from build123d import *

# Parameters (mm, degrees)
SKETCH1_R           = 1.5
BOSS_EXTRUDE1_DEPTH = 1.75
BOSS_EXTRUDE2_DEPTH = 3
BOSS_EXTRUDE3_DEPTH = 0.5
SKETCH4_R           = 0.26
CUT_EXTRUDE1_DEPTH  = 42.78890403


with BuildPart() as part:
    # Sketch1 → Boss-Extrude1 (new body)
    with BuildSketch(Plane(origin=(0, 0, 0), x_dir=(1, 0, 0), z_dir=(0, 1, 0))):
        with BuildLine():
            Line((-18, 20), (18, 20))
            ThreePointArc((18, 20), (19.414213562, 19.414213562), (20, 18))
            Line((20, 18), (20, -18))
            ThreePointArc((20, -18), (19.414213562, -19.414213562), (18, -20))
            Line((18, -20), (-18, -20))
            ThreePointArc((-18, -20), (-19.414213562, -19.414213562), (-20, -18))
            Line((-20, -18), (-20, 18))
            ThreePointArc((-20, 18), (-19.414213562, 19.414213562), (-18, 20))
        make_face()
        with Locations(Location((-15.25, 15.25, 0), (0, 0, 270))):
            Circle(SKETCH1_R, mode=Mode.SUBTRACT)
        with Locations(Location((15.25, 15.25, 0), (0, 0, 270))):
            Circle(SKETCH1_R, mode=Mode.SUBTRACT)
        with Locations(Location((15.25, -15.25, 0), (0, 0, 270))):
            Circle(SKETCH1_R, mode=Mode.SUBTRACT)
        with Locations(Location((-15.25, -15.25, 0), (0, 0, 270))):
            Circle(SKETCH1_R, mode=Mode.SUBTRACT)
    extrude(amount=BOSS_EXTRUDE1_DEPTH)

    # Sketch2 → Boss-Extrude2 (add)
    with BuildSketch(Plane.XY.offset(20)):
        with BuildLine():
            Line((7.26, 1.75), (7.26, 2.78))
            ThreePointArc((7.26, 2.78), (7.318578644, 2.921421356), (7.46, 2.98))
            Line((7.46, 2.98), (7.705, 2.98))
            ThreePointArc((7.705, 2.98), (7.846421356, 3.038578644), (7.905, 3.18))
            Line((7.905, 3.18), (7.905, 3.55))
            ThreePointArc((7.905, 3.55), (7.963578644, 3.691421356), (8.105, 3.75))
            Line((8.105, 3.75), (10.415, 3.75))
            ThreePointArc((10.415, 3.75), (10.556421356, 3.691421356), (10.615, 3.55))
            Line((10.615, 3.55), (10.615, 3.18))
            ThreePointArc((10.615, 3.18), (10.673578644, 3.038578644), (10.815, 2.98))
            Line((10.815, 2.98), (11.06, 2.98))
            ThreePointArc((11.06, 2.98), (11.201421356, 2.921421356), (11.26, 2.78))
            Line((11.26, 2.78), (11.26, 1.75))
            Line((11.26, 1.75), (7.26, 1.75))
        make_face()
        with BuildLine():
            Line((7.36, 1.85), (7.36, 2.78))
            ThreePointArc((7.36, 2.78), (7.389289322, 2.850710678), (7.46, 2.88))
            Line((7.46, 2.88), (7.705, 2.88))
            ThreePointArc((7.705, 2.88), (7.917132034, 2.967867966), (8.005, 3.18))
            Line((8.005, 3.18), (8.005, 3.55))
            ThreePointArc((8.005, 3.55), (8.034289322, 3.620710678), (8.105, 3.65))
            Line((8.105, 3.65), (10.415, 3.65))
            ThreePointArc((10.415, 3.65), (10.485710678, 3.620710678), (10.515, 3.55))
            Line((10.515, 3.55), (10.515, 3.18))
            ThreePointArc((10.515, 3.18), (10.602867966, 2.967867966), (10.815, 2.88))
            Line((10.815, 2.88), (11.06, 2.88))
            ThreePointArc((11.06, 2.88), (11.130710678, 2.850710678), (11.16, 2.78))
            Line((11.16, 2.78), (11.16, 1.85))
            Line((11.16, 1.85), (7.36, 1.85))
        make_face(mode=Mode.SUBTRACT)
    extrude(amount=-BOSS_EXTRUDE2_DEPTH)

    # Sketch3 → Boss-Extrude3 (add)
    with BuildSketch(Plane(origin=(0, 0, 17), x_dir=(-1, 0, 0), z_dir=(0, 0, -1))):
        with BuildLine():
            Line((-11.26, 1.75), (-7.26, 1.75))
            Line((-7.26, 1.75), (-7.26, 2.78))
            ThreePointArc((-7.26, 2.78), (-7.318578644, 2.921421356), (-7.46, 2.98))
            Line((-7.46, 2.98), (-7.705, 2.98))
            ThreePointArc((-7.705, 2.98), (-7.846421356, 3.038578644), (-7.905, 3.18))
            Line((-7.905, 3.18), (-7.905, 3.55))
            ThreePointArc((-7.905, 3.55), (-7.963578644, 3.691421356), (-8.105, 3.75))
            Line((-8.105, 3.75), (-10.415, 3.75))
            ThreePointArc((-10.415, 3.75), (-10.556421356, 3.691421356), (-10.615, 3.55))
            Line((-10.615, 3.55), (-10.615, 3.18))
            ThreePointArc((-10.615, 3.18), (-10.673578644, 3.038578644), (-10.815, 2.98))
            Line((-10.815, 2.98), (-11.06, 2.98))
            ThreePointArc((-11.06, 2.98), (-11.201421356, 2.921421356), (-11.26, 2.78))
            Line((-11.26, 2.78), (-11.26, 1.75))
        make_face()
    extrude(amount=BOSS_EXTRUDE3_DEPTH)

    # Sketch4 → Cut-Extrude1 (cut, through all)
    with BuildSketch(Plane(origin=(0, 0, 16.5), x_dir=(-1, 0, 0), z_dir=(0, 0, -1))):
        with Locations((-10.2, 2.87)):
            Circle(SKETCH4_R)
        with Locations((-9.3, 2.87)):
            Circle(SKETCH4_R)
        with Locations((-8.4, 2.87)):
            Circle(SKETCH4_R)
    extrude(amount=-CUT_EXTRUDE1_DEPTH, mode=Mode.SUBTRACT)


solid = part.part
Source: CAD feature listing. Evaluate the final solid. Frame: model axes, mm. A direction names the side the tool comes from. Coordinates: 2 decimals unless noted, no trailing zeros. Order: outer loops, then holes, each group sorted by start corner. A loop starts at its lowest first (then second) coordinate and runs counter-clockwise, first axis right, second up. Notation, with made-up numbers: M 59.25,-26 L 76.25,-26 A11 cw 76.25,-12 Z; hole C 4,16.25 d10. An arc over 180 degrees is marked long. Write each question's results on one line, items separated by ' | '. Start each with the question number.
1. Section D-D, the plane x = 3.5. Return the cut outline in (y, z), then the cut area to 3 significant figures.
2. Draft query along Y for faces 1 (the face through (-20, 1, 0)), 2 (the face through (0, 0, 0)), 3 (the face through (9, 1.85, 19)). Return one class per face: +Y half, -Y half, draft (parallel to the pull), parting line (faces both ways), or undercut.
3. Section B-B, the plane z = -15.25. Return the cut outline in (x, y).
4. Reachability of faces 4 (the face through (9, 2, 16.5)), 5 (the face through (-15.18, 0.86, -16.75)) from +Z, -Z, +X, -X, +Y, -Y: full face, straight path, thin tool, end or side. Return the list, or none.
5. Section C-C, the plane y = 0.8. Return the cut outline in (x, z), then the cut area to 3 significant figures.
6. Section A-A, the plane x = 15.25. Return the cut outline in (y, z).
7. Material intervals for L1, parallel to X at y = 1.05, z = 15.25; L2, parallel to Y at x = 9.3, z = 16.6; L3, parallel to Y at x = 10, z = 6.5, sorted ascending.
8. Pin query (flat end, axial travel): pin 1 (1 mm diameter, centred on x = 9, y = 2.5, fed in from -Z); pin 2 (3 mm diameter, centred on x = -13.5, z = -6.5, fed in from -Y); pin 3 (0.8 mm diameter, centred on y = 2.5, z = 19, fed in from -X); pin 4 (8 mm diameter, centred on x = -14, z = 3.5, fed in from +Y). Return the tip coordinate at first contact, or that it passes through.
Solution:
1) outline: M 0,-20 L 1.75,-20 L 1.75,20 L 0,20 Z | area: 70.0 mm²
2) face 1: draft | face 2: -Y half | face 3: undercut
3) outline: M -20,0 L -16.75,0 L -16.75,1.75 L -20,1.75 Z; M -13.75,0 L 13.75,0 L 13.75,1.75 L -13.75,1.75 Z; M 16.75,0 L 20,0 L 20,1.75 L 16.75,1.75 Z
4) face 4: -Z, +X, -X, +Y | face 5: +Y, -Y
5) outline: M -20,-18 A2 ccw -18,-20 L 18,-20 A2 ccw 20,-18 L 20,18 A2 ccw 18,20 L -18,20 A2 ccw -20,18 Z; hole C -15.25,-15.25 d3; hole C -15.25,15.25 d3; hole C 15.25,-15.25 d3; hole C 15.25,15.25 d3 | area: 1,570 mm²
6) outline: M 0,-20 L 1.75,-20 L 1.75,-16.75 L 0,-16.75 Z; M 0,-13.75 L 1.75,-13.75 L 1.75,13.75 L 0,13.75 Z; M 0,16.75 L 1.75,16.75 L 1.75,20 L 0,20 Z
7) L1: -20 to -16.75, -13.75 to 13.75, 16.75 to 20 | L2: 0 to 2.61, 3.13 to 3.75 | L3: 0 to 1.75
8) pin 1: z = 16.5 | pin 2: y = 0 | pin 3: x = 7.26 | pin 4: y = 1.75
